from build123d import *

# Parameters (mm, degrees)
F0_R          = 3
F1_DEPTH      = 5
F0_R_2        = 1.55
F2_DEPTH      = 3
F0_W          = 10
F0_H          = 10
F3_DEPTH      = 5
F3_DEPTH_BACK = 20
F4_DEPTH      = 48
F4_DEPTH_BACK = 20
F5_DEPTH      = 58


with BuildPart() as f1:
    # F0 (on Top) → F1 (new body)
    with BuildSketch(Plane.XY):
        with BuildLine():
            ThreePointArc((-9.2330926563, -5), (-10.5, 0), (-9.2330926563, 5))
            Line((-9.2330926563, 5), (-25, 5))
            Line((-25, 5), (-25, -5))
            Line((-25, -5), (-9.2330926563, -5))
        make_face()
        with Locations((-17.5, 0)):
            Circle(F0_R, mode=Mode.SUBTRACT)
    extrude(amount=F1_DEPTH)

    # F0 (on Top) → F2, piece 4 (join)
    with BuildSketch(Plane.XY):
        with Locations((-17.5, 0)):
            Circle(F0_R)
        with Locations((-17.5, 0)):
            Circle(F0_R_2, mode=Mode.SUBTRACT)
    extrude(amount=F2_DEPTH)

    # F0 (on Top) → F3, piece 4 (join, two sides)
    with BuildSketch(Plane.XY) as f3_4_sk:
        with Locations((-30, 0)):
            Rectangle(F0_W, F0_H)
    extrude(amount=F3_DEPTH)
    extrude(f3_4_sk.sketch, amount=-F3_DEPTH_BACK)



with BuildPart() as f1b:
    # F0 (on Top) → F1, piece 2 (new body)
    with BuildSketch(Plane.XY):
        with BuildLine():
            ThreePointArc((-5, 9.2330926563), (0, 10.5), (5, 9.2330926563))
            Line((5, 9.2330926563), (5, 25))
            Line((5, 25), (-5, 25))
            Line((-5, 25), (-5, 9.2330926563))
        make_face()
        with Locations((0, 17.5)):
            Circle(F0_R, mode=Mode.SUBTRACT)
    extrude(amount=F1_DEPTH)

    # F0 (on Top) → F2 (join)
    with BuildSketch(Plane.XY):
        with Locations((0, 17.5)):
            Circle(F0_R)
        with Locations((0, 17.5)):
            Circle(F0_R_2, mode=Mode.SUBTRACT)
    extrude(amount=F2_DEPTH)

    # F0 (on Top) → F3 (join, two sides)
    with BuildSketch(Plane.XY) as f3_sk:
        with Locations((0, 30)):
            Rectangle(F0_W, F0_H)
    extrude(amount=F3_DEPTH)
    extrude(f3_sk.sketch, amount=-F3_DEPTH_BACK)


with BuildPart() as f1c:
    # F0 (on Top) → F1, piece 3 (new body)
    with BuildSketch(Plane.XY):
        with BuildLine():
            Line((25, 5), (9.2330926563, 5))
            ThreePointArc((9.2330926563, 5), (10.1783464495, 2.5790043727), (10.5, 0))
            ThreePointArc((10.5, 0), (10.1783464495, -2.5790043727), (9.2330926563, -5))
            Line((9.2330926563, -5), (25, -5))
            Line((25, -5), (25, 5))
        make_face()
        with Locations((17.5, 0)):
            Circle(F0_R, mode=Mode.SUBTRACT)
    extrude(amount=F1_DEPTH)

    # F0 (on Top) → F2, piece 2 (join)
    with BuildSketch(Plane.XY):
        with Locations((17.5, 0)):
            Circle(F0_R)
        with Locations((17.5, 0)):
            Circle(F0_R_2, mode=Mode.SUBTRACT)
    extrude(amount=F2_DEPTH)

    # F0 (on Top) → F3, piece 2 (join, two sides)
    with BuildSketch(Plane.XY) as f3_2_sk:
        with Locations((30, 0)):
            Rectangle(F0_W, F0_H)
    extrude(amount=F3_DEPTH)
    extrude(f3_2_sk.sketch, amount=-F3_DEPTH_BACK)


with BuildPart() as f1d:
    # F0 (on Top) → F1, piece 4 (new body)
    with BuildSketch(Plane.XY):
        with BuildLine():
            Line((5, -25), (5, -9.2330926563))
            ThreePointArc((5, -9.2330926563), (0, -10.5), (-5, -9.2330926563))
            Line((-5, -9.2330926563), (-5, -25))
            Line((-5, -25), (5, -25))
        make_face()
        with Locations((0, -17.5)):
            Circle(F0_R, mode=Mode.SUBTRACT)
    extrude(amount=F1_DEPTH)

    # F0 (on Top) → F2, piece 3 (join)
    with BuildSketch(Plane.XY):
        with Locations((0, -17.5)):
            Circle(F0_R)
        with Locations((0, -17.5)):
            Circle(F0_R_2, mode=Mode.SUBTRACT)
    extrude(amount=F2_DEPTH)

    # F0 (on Top) → F3, piece 3 (join, two sides)
    with BuildSketch(Plane.XY) as f3_3_sk:
        with Locations((0, -30)):
            Rectangle(F0_W, F0_H)
    extrude(amount=F3_DEPTH)
    extrude(f3_3_sk.sketch, amount=-F3_DEPTH_BACK)


with BuildPart() as f1_1:
    add(f1.part)

    add(f1b.part)  # F4 merges F1b

    add(f1c.part)  # F4 merges F1c

    add(f1d.part)  # F4 merges F1d
    # F0 (on Top) → F4 (join, two sides)
    with BuildSketch(Plane.XY) as f4_sk:
        with BuildLine():
            Line((-5, -9.2330926563), (-5, -5.5229068433))
            ThreePointArc((-5, -5.5229068433), (-5.2679455198, -5.2679455198), (-5.5229068433, -5))
            Line((-5.5229068433, -5), (-9.2330926563, -5))
            ThreePointArc((-9.2330926563, -5), (-7.4246212025, -7.4246212025), (-5, -9.2330926563))
        make_face()
        with BuildLine():
            ThreePointArc((-5.5229068433, -5), (-7.45, 0), (-5.5229068433, 5))
            Line((-5.5229068433, 5), (-9.2330926563, 5))
            ThreePointArc((-9.2330926563, 5), (-10.5, 0), (-9.2330926563, -5))
            Line((-9.2330926563, -5), (-5.5229068433, -5))
        make_face()
        with BuildLine():
            Line((-5, -5), (-5, 5))
            Line((-5, 5), (-5.5229068433, 5))
            ThreePointArc((-5.5229068433, 5), (-7.45, 0), (-5.5229068433, -5))
            Line((-5.5229068433, -5), (-5, -5))
        make_face()
        with BuildLine():
            ThreePointArc((-5.5229068433, -5), (-5.2679455198, -5.2679455198), (-5, -5.5229068433))
            Line((-5, -5.5229068433), (-5, -5))
            Line((-5, -5), (-5.5229068433, -5))
        make_face()
        with BuildLine():
            ThreePointArc((-5, -5.5229068433), (0, -7.45), (5, -5.5229068433))
            Line((5, -5.5229068433), (5, -5))
            Line((5, -5), (-5, -5))
            Line((-5, -5), (-5, -5.5229068433))
        make_face()
        with BuildLine():
            Line((5, -9.2330926563), (5, -5.5229068433))
            ThreePointArc((5, -5.5229068433), (0, -7.45), (-5, -5.5229068433))
            Line((-5, -5.5229068433), (-5, -9.2330926563))
            ThreePointArc((-5, -9.2330926563), (0, -10.5), (5, -9.2330926563))
        make_face()
        Rectangle(F0_W, F0_H)
        with BuildLine():
            ThreePointArc((5.5229068433, -5), (6.9515522001, -2.6792577346), (7.45, 0))
            ThreePointArc((7.45, 0), (6.9515522001, 2.6792577346), (5.5229068433, 5))
            Line((5.5229068433, 5), (5, 5))
            Line((5, 5), (5, -5))
            Line((5, -5), (5.5229068433, -5))
        make_face()
        with BuildLine():
            Line((9.2330926563, -5), (5.5229068433, -5))
            ThreePointArc((5.5229068433, -5), (5.2679455198, -5.2679455198), (5, -5.5229068433))
            Line((5, -5.5229068433), (5, -9.2330926563))
            ThreePointArc((5, -9.2330926563), (7.4246212025, -7.4246212025), (9.2330926563, -5))
        make_face()
        with BuildLine():
            ThreePointArc((5, -5.5229068433), (5.2679455198, -5.2679455198), (5.5229068433, -5))
            Line((5.5229068433, -5), (5, -5))
            Line((5, -5), (5, -5.5229068433))
        make_face()
        with BuildLine():
            ThreePointArc((5.5229068433, 5), (6.9515522001, 2.6792577346), (7.45, 0))
            ThreePointArc((7.45, 0), (6.9515522001, -2.6792577346), (5.5229068433, -5))
            Line((5.5229068433, -5), (9.2330926563, -5))
            ThreePointArc((9.2330926563, -5), (10.1783464495, -2.5790043727), (10.5, 0))
            ThreePointArc((10.5, 0), (10.1783464495, 2.5790043727), (9.2330926563, 5))
            Line((9.2330926563, 5), (5.5229068433, 5))
        make_face()
        with BuildLine():
            Line((5, 5), (5.5229068433, 5))
            ThreePointArc((5.5229068433, 5), (5.2679455198, 5.2679455198), (5, 5.5229068433))
            Line((5, 5.5229068433), (5, 5))
        make_face()
        with BuildLine():
            ThreePointArc((5, 5.5229068433), (5.2679455198, 5.2679455198), (5.5229068433, 5))
            Line((5.5229068433, 5), (9.2330926563, 5))
            ThreePointArc((9.2330926563, 5), (7.4246212025, 7.4246212025), (5, 9.2330926563))
            Line((5, 9.2330926563), (5, 5.5229068433))
        make_face()
        with BuildLine():
            Line((5, 5), (5, 5.5229068433))
            ThreePointArc((5, 5.5229068433), (0, 7.45), (-5, 5.5229068433))
            Line((-5, 5.5229068433), (-5, 5))
            Line((-5, 5), (5, 5))
        make_face()
        with BuildLine():
            ThreePointArc((-5, 5.5229068433), (0, 7.45), (5, 5.5229068433))
            Line((5, 5.5229068433), (5, 9.2330926563))
            ThreePointArc((5, 9.2330926563), (0, 10.5), (-5, 9.2330926563))
            Line((-5, 9.2330926563), (-5, 5.5229068433))
        make_face()
        with BuildLine():
            ThreePointArc((-5.5229068433, 5), (-5.2679455198, 5.2679455198), (-5, 5.5229068433))
            Line((-5, 5.5229068433), (-5, 9.2330926563))
            ThreePointArc((-5, 9.2330926563), (-7.4246212025, 7.4246212025), (-9.2330926563, 5))
            Line((-9.2330926563, 5), (-5.5229068433, 5))
        make_face()
        with BuildLine():
            Line((-5, 5), (-5, 5.5229068433))
            ThreePointArc((-5, 5.5229068433), (-5.2679455198, 5.2679455198), (-5.5229068433, 5))
            Line((-5.5229068433, 5), (-5, 5))
        make_face()
    extrude(amount=F4_DEPTH)
    extrude(f4_sk.sketch, amount=-F4_DEPTH_BACK)

    # F0 (on Top) → F5 (join)
    with BuildSketch(Plane.XY):
        Rectangle(F0_W, F0_H)
        with BuildLine():
            Line((-5, -5), (-5, 5))
            Line((-5, 5), (-5.5229068433, 5))
            ThreePointArc((-5.5229068433, 5), (-7.45, 0), (-5.5229068433, -5))
            Line((-5.5229068433, -5), (-5, -5))
        make_face()
        with BuildLine():
            Line((5, 5), (5, 5.5229068433))
            ThreePointArc((5, 5.5229068433), (0, 7.45), (-5, 5.5229068433))
            Line((-5, 5.5229068433), (-5, 5))
            Line((-5, 5), (5, 5))
        make_face()
        with BuildLine():
            ThreePointArc((5.5229068433, -5), (6.9515522001, -2.6792577346), (7.45, 0))
            ThreePointArc((7.45, 0), (6.9515522001, 2.6792577346), (5.5229068433, 5))
            Line((5.5229068433, 5), (5, 5))
            Line((5, 5), (5, -5))
            Line((5, -5), (5.5229068433, -5))
        make_face()
        with BuildLine():
            ThreePointArc((-5, -5.5229068433), (0, -7.45), (5, -5.5229068433))
            Line((5, -5.5229068433), (5, -5))
            Line((5, -5), (-5, -5))
            Line((-5, -5), (-5, -5.5229068433))
        make_face()
        with BuildLine():
            ThreePointArc((-5.5229068433, -5), (-5.2679455198, -5.2679455198), (-5, -5.5229068433))
            Line((-5, -5.5229068433), (-5, -5))
            Line((-5, -5), (-5.5229068433, -5))
        make_face()
        with BuildLine():
            ThreePointArc((5, -5.5229068433), (5.2679455198, -5.2679455198), (5.5229068433, -5))
            Line((5.5229068433, -5), (5, -5))
            Line((5, -5), (5, -5.5229068433))
        make_face()
        with BuildLine():
            Line((5, 5), (5.5229068433, 5))
            ThreePointArc((5.5229068433, 5), (5.2679455198, 5.2679455198), (5, 5.5229068433))
            Line((5, 5.5229068433), (5, 5))
        make_face()
        with BuildLine():
            Line((-5, 5), (-5, 5.5229068433))
            ThreePointArc((-5, 5.5229068433), (-5.2679455198, 5.2679455198), (-5.5229068433, 5))
            Line((-5.5229068433, 5), (-5, 5))
        make_face()
    extrude(amount=F5_DEPTH)


solid = f1_1.part
Read the model definition and answer for the solid it produces. Units are mm, in the model's axes. A direction names the side the tool comes from. Coordinates: 2 decimals unless noted, no trailing zeros. Order: outer loops, then holes, each group sorted by start corner. A loop starts at its lowest first (then second) coordinate and runs counter-clockwise, first axis right, second up. Notation, with made-up numbers: (-32, 35.5) -> (-20, 35.5) arc R12 ccw to (-20, 49.5) -> close; hole circle Ø4 at (20.5, 69). An arc over 180 degrees is marked (long way). Answer as a JSON object with one key per item and string values.
1) Consider line 1 along Y through (x, z) = (0, 4); line 2 along X through (y, z) = (4, -12); line 3 along X through (y, z) = (-3, -3.5). Determine where each line is inside the solid, lowest interval first. Write a range as from..to.
Model answer:
{"line 1": "y = -35..-20.5, -14.5..14.5, 20.5..35", "line 2": "x = -35..-25, -9.71..9.71, 25..35", "line 3": "x = -35..-25, -10.06..10.06, 25..35"}
2) Each of these flat-tipped pins is pushed along its axis until it touches: pin 1 (4 mm diameter, centred on x = -17.5, y = 0, fed in from -Z); pin 2 (7.5 mm diameter, centred on y = -27, z = -6, fed in from +X); pin 3 (20 mm diameter, centred on x = 22.5, z = -1.5, fed in from -Y). Where does it stop, or does it pass through?
Model answer:
{"pin 1": "stops at z = 0", "pin 2": "stops at x = 5", "pin 3": "stops at y = -5"}
3) A cutting plane is placed at D-D, the plane z = 40. Determine the outline of the cut face in (x, y).
Model answer:
{"outline": "circle Ø21 at (0, 0)"}
4) A cutting plane is placed at C-C, the plane z = -13. Determine the outline of the cut face in (x, y), plus the area to 3 significant figures.
Model answer:
{"outline": "(-35, -5) -> (-25, -5) -> (-25, 5) -> (-35, 5) -> close; circle Ø21 at (0, 0); (-5, -35) -> (5, -35) -> (5, -25) -> (-5, -25) -> close; (-5, 25) -> (5, 25) -> (5, 35) -> (-5, 35) -> close; (25, -5) -> (35, -5) -> (35, 5) -> (25, 5) -> close", "area": "746 mm²"}
5) A cutting plane is placed at A-A, the plane x = 17.5. Determine the outline of the cut face in (y, z), plus the area to 3 significant figures.
Model answer:
{"outline": "(-5, 0) -> (-1.55, 0) -> (-1.55, 3) -> (-3, 3) -> (-3, 5) -> (-5, 5) -> close; (1.55, 0) -> (5, 0) -> (5, 5) -> (3, 5) -> (3, 3) -> (1.55, 3) -> close", "area": "28.7 mm²"}
6) The mould has two halves that part along X. Classify faces 4 (the face through (0, 35, -7)), 5 (the face through (35, 0, -7)), 6 (the face through (-0.202, -15.963, 1.479)), 7 (the face through (-20.5, 0.1, 4)): released by +X, released by -X, zero draft, split by the parting line, or undercut.
Model answer:
{"face 4": "zero draft", "face 5": "released by +X", "face 6": "undercut", "face 7": "undercut"}
7) A tool of negligible diameter and unlimited length cuts with its end or side. For faces 1 (the face through (25, 0, -10)), 2 (the face through (0, 25, -10)), 3 (the face through (-16, -1, 3)), from which of +Z, -Z, +X, -X, +Y, -Y can it reach the whole face along a straight path? Write none if from no direction.
Model answer:
{"face 1": "-Z, +Y, -Y", "face 2": "-Z, +X, -X", "face 3": "+Z"}
